```python
from build123d import *

# Parameters (mm, degrees)
BOSS_EXTRUDE1_DEPTH = 5
SKETCH2_R           = 4.85
BOSS_EXTRUDE2_DEPTH = 8
SKETCH3_R           = 4.85
BOSS_EXTRUDE3_DEPTH = 8
CHAMFER1_SIZE       = 0.5
SKETCH4_R           = 2.5
CUT_EXTRUDE1_DEPTH  = 22


with BuildPart() as part:
    # Sketch1 → Boss-Extrude1 (new body)
    with BuildSketch(Plane(origin=(0, 0, 0), x_dir=(1, 0, 0), z_dir=(0, 1, 0))):
        Polygon((4.041451884, -7), (8.082903769, 0), (4.041451884, 7), (-4.041451884, 7), (-8.082903769, 0), (-4.041451884, -7), align=None)
    extrude(amount=BOSS_EXTRUDE1_DEPTH)

    # Sketch2 → Boss-Extrude2 (add)
    with BuildSketch(Plane(origin=(0, 5, 0), x_dir=(1, 0, 0), z_dir=(0, 1, 0))):
        Circle(SKETCH2_R)
    extrude(amount=BOSS_EXTRUDE2_DEPTH)

    # Sketch3 → Boss-Extrude3 (add)
    with BuildSketch(Plane.XZ):
        Circle(SKETCH3_R)
    extrude(amount=BOSS_EXTRUDE3_DEPTH)

    # Chamfer1
    chamfer1_edges = [part.edges().sort_by_distance(p)[0] for p in [
        (-4.85, 13, 0),
        (-4.85, -8, 0),
    ]]
    chamfer(chamfer1_edges, length=CHAMFER1_SIZE)

    # Sketch4 → Cut-Extrude1 (cut, through all)
    with BuildSketch(Plane(origin=(0, 13, 0), x_dir=(1, 0, 0), z_dir=(0, 1, 0))):
        Circle(SKETCH4_R)
    extrude(amount=-CUT_EXTRUDE1_DEPTH, mode=Mode.SUBTRACT)


solid = part.part
```
Read the model definition and answer for the solid it produces. Units are mm, in the model's axes. A direction names the side the tool comes from. Coordinates: 2 decimals unless noted, no trailing zeros. Loops run counter-clockwise (first coordinate to the right, second up) from the corner with the lowest first, then second, coordinate; pieces in that order, holes last. Notation, with made-up numbers: (1.5, -14) - (9.5, -14) arc R12 cw to (9.5, 2) - close; hole circle Ø1 at (58, -15.75). An arc over 180 degrees is marked (long way). Answer in a Markdown table with one row per item.
1. Straight lines are drawn through the part: line 1 (Z direction, x = 0, y = 5.5); line 2 (Y direction, x = 7, z = -0.75); line 3 (X direction, y = 2.25, z = -1.75). For each, find the intervals that lie inside material, in ascending order.
Conclusion:
| item | result |
|---|---|
| line 1 | z = -4.85 to -2.5, 2.5 to 4.85 |
| line 2 | y = 0 to 5 |
| line 3 | x = -7.07 to -1.79, 1.79 to 7.07 |
2. Given pin 1 (3 mm diameter, centred on x = 0, z = 0, fed in from +Y); pin 2 (8 mm diameter, centred on y = -0.5, z = -4, fed in from +X); pin 3 (2 mm diameter, centred on x = -4.5, y = -1.5, fed in from -Z); pin 4 (2 mm diameter, centred on x = 2, y = 9.5, fed in from +Z), each flat-ended and moving along its own axis, determine where each tip first touches the part or whether it passes through.
Conclusion:
| item | result |
|---|---|
| pin 1 | passes through |
| pin 2 | stops at x = 8.06 |
| pin 3 | stops at z = -3.36 |
| pin 4 | stops at z = 4.75 |
3. Find section C-C, the plane x = -7. Write down the section's boundary in (y, z), then the cut area to 3 significant figures.
Conclusion:
| item | result |
|---|---|
| outline | (0, -1.88) - (5, -1.88) - (5, 1.88) - (0, 1.88) - close |
| area | 18.8 mm² |
4. Determine the mould class of faces 4 (the face through (4.626, 8.698, -1.457)), 5 (the face through (2, -8, -2)), 6 (the face through (6.034, 2.465, 3.549)), 7 (the face through (-0.54, 2.65, 2.44)) for opening direction Z: +Z half, -Z half, draft (parallel to the pull), parting line (faces both ways), or undercut.
Conclusion:
| item | result |
|---|---|
| face 4 | parting line |
| face 5 | draft |
| face 6 | +Z half |
| face 7 | undercut |
5. Find section D-D, the plane z = 5.25. Write down the section's boundary in (x, y), then the cut area to 3 significant figures.
Conclusion:
| item | result |
|---|---|
| outline | (-5.05, 0) - (5.05, 0) - (5.05, 5) - (-5.05, 5) - close |
| area | 50.5 mm² |
6. Which of the six approach directions +Z, -Z, +X, -X, +Y, -Y give full straight-line access (tool end or side, diameter ignored) to faces 1 (the face through (2, 5, -5)), 2 (the face through (4.626, -3.698, 1.457)), 3 (the face through (0, 2, 7))?
Conclusion:
| item | result |
|---|---|
| face 1 | +Y |
| face 2 | -Y |
| face 3 | +Z, +X, -X, +Y, -Y |
7. Find section B-B, the plane y = 2.25. Write down the section's boundary in (x, z), then the cut area to 3 significant figures.
Conclusion:
| item | result |
|---|---|
| outline | (-8.08, 0) - (-4.04, -7) - (4.04, -7) - (8.08, 0) - (4.04, 7) - (-4.04, 7) - close; hole circle Ø5 at (0, 0) |
| area | 150 mm² |
8. Find section A-A, the plane x = 0. Write down the section's boundary in (y, z), then the cut area to 3 significant figures.
Conclusion:
| item | result |
|---|---|
| outline | (-8, -4.35) - (-7.5, -4.85) - (0, -4.85) - (0, -7) - (5, -7) - (5, -4.85) - (12.5, -4.85) - (13, -4.35) - (13, -2.5) - (-8, -2.5) - close; (-8, 2.5) - (13, 2.5) - (13, 4.35) - (12.5, 4.85) - (5, 4.85) - (5, 7) - (0, 7) - (0, 4.85) - (-7.5, 4.85) - (-8, 4.35) - close |
| area | 120 mm² |
